from build123d import *

# Parameters (mm, degrees)
SKETCH_1_W                   = 80
SKETCH_1_H                   = 100
EXTRUDE_1_DEPTH              = 11
SKETCH_7_W                   = 15
SKETCH_7_H                   = 30
CUT_EXTRUDE_1_DEPTH          = 16
HOLE_WIZARD_M4_1_D           = 3.3
HOLE_WIZARD_M4_1_CSINK_D     = 4.05
HOLE_WIZARD_M4_1_CSINK_ANGLE = 90
FILLET_1_R                   = 20
FILLET_2_R                   = 2
SKETCH_9_W                   = 6
SKETCH_9_H                   = 35
CUT_EXTRUDE_2_DEPTH          = 11
SKETCH_11_R                  = 3
CUT_EXTRUDE_4_DEPTH          = 15
SKETCH_12_R                  = 3.43
CUT_EXTRUDE_5_DEPTH          = 3.9
CUT_EXTRUDE_6_DEPTH          = 5.4
CUT_EXTRUDE_7_DEPTH          = 14
SKETCH_15_R                  = 1.9
CUT_EXTRUDE_8_DEPTH          = 14
FILLET_4_R                   = 0.12
FILLET_5_R                   = 1


with BuildPart() as part:
    # 草图1 → 凸台-拉伸1 (new body)
    with BuildSketch(Plane.XY):
        Rectangle(SKETCH_1_W, SKETCH_1_H)
    extrude(amount=EXTRUDE_1_DEPTH)

    # 草图7 → 切除-拉伸1 (cut)
    with BuildSketch(Plane.XY.offset(11)):
        with Locations((0, 35)):
            Rectangle(SKETCH_7_W, SKETCH_7_H)
    extrude(amount=-CUT_EXTRUDE_1_DEPTH, mode=Mode.SUBTRACT)

    # M4 螺纹孔1 (through all)
    with Locations(Plane(origin=(13.5, 24.75, 0), x_dir=(-1, 0, 0), z_dir=(0, 0, -1))):
        with Locations((0, 0), (27, 0), (41.5, -49.5), (-14.5, -49.5)):
            CounterSinkHole(HOLE_WIZARD_M4_1_D / 2, HOLE_WIZARD_M4_1_CSINK_D / 2, counter_sink_angle=HOLE_WIZARD_M4_1_CSINK_ANGLE)

    # 圆角1
    fillet_1_edges = [part.edges().sort_by_distance(p)[0] for p in [
        (-40, 50, 5.5),
        (40, 50, 5.5),
    ]]
    fillet(fillet_1_edges, radius=FILLET_1_R)

    # 圆角2
    fillet_2_edges = [part.edges().sort_by_distance(p)[0] for p in [
        (-7.5, 20, 5.5),
        (-7.5, 50, 5.5),
        (7.5, 50, 5.5),
        (7.5, 20, 5.5),
        (40, -50, 5.5),
        (-40, -50, 5.5),
    ]]
    fillet(fillet_2_edges, radius=FILLET_2_R)

    # 草图9 → 切除-拉伸2 (cut)
    with BuildSketch(Plane.XY):
        with Locations((37, 0)):
            Rectangle(SKETCH_9_W, SKETCH_9_H)
        with Locations((-37, 0)):
            Rectangle(SKETCH_9_W, SKETCH_9_H)
    extrude(amount=CUT_EXTRUDE_2_DEPTH, mode=Mode.SUBTRACT)

    # 草图11 → 切除-拉伸4 (cut)
    with BuildSketch(Plane.XY):
        with Locations((-22.273863607, 38.273863607)):
            Circle(SKETCH_11_R)
        with Locations((22.273863607, 38.273863607)):
            Circle(SKETCH_11_R)
        with Locations((22.273863607, -6.273863607)):
            Circle(SKETCH_11_R)
        with Locations((-22.273863607, -6.273863607)):
            Circle(SKETCH_11_R)
    extrude(amount=CUT_EXTRUDE_4_DEPTH, mode=Mode.SUBTRACT)

    # 草图12 → 切除-拉伸5 (cut)
    with BuildSketch(Plane.XY):
        with Locations((13.5, 24.75)):
            Circle(SKETCH_12_R)
        with Locations((28, -24.75)):
            Circle(SKETCH_12_R)
        with Locations(Location((-28, -24.75, 0), (0, 0, 180))):
            Circle(SKETCH_12_R)
        with Locations(Location((-13.5, 24.75, 0), (0, 0, 180))):
            Circle(SKETCH_12_R)
    extrude(amount=CUT_EXTRUDE_5_DEPTH, mode=Mode.SUBTRACT)

    # 草图13 → 切除-拉伸6 (cut)
    with BuildSketch(Plane.XY.offset(11)):
        Polygon((-19.42752678, 33.343863607), (-16.581189953, 38.273863607), (-19.42752678, 43.203863607), (-25.120200434, 43.203863607), (-27.966537262, 38.273863607), (-25.120200434, 33.343863607), align=None)
        Polygon((-19.42752678, -11.203863607), (-16.581189953, -6.273863607), (-19.42752678, -1.343863607), (-25.120200434, -1.343863607), (-27.966537262, -6.273863607), (-25.120200434, -11.203863607), align=None)
        Polygon((25.120200434, -11.203863607), (19.42752678, -11.203863607), (16.581189953, -6.273863607), (19.42752678, -1.343863607), (25.120200434, -1.343863607), (27.966537262, -6.273863607), align=None)
        Polygon((25.120200434, 33.343863607), (19.42752678, 33.343863607), (16.581189953, 38.273863607), (19.42752678, 43.203863607), (25.120200434, 43.203863607), (27.966537262, 38.273863607), align=None)
    extrude(amount=-CUT_EXTRUDE_6_DEPTH, mode=Mode.SUBTRACT)

    # 草图14 → 切除-拉伸7 (cut)
    with BuildSketch(Plane(origin=(0, 0, 0), x_dir=(-1, 0, 0), z_dir=(0, 0, -1))):
        with BuildLine():
            Line((-42.281489137, -24.75), (-32.43, -24.75))
            ThreePointArc((-32.43, -24.75), (-32.229391744, -26.068008147), (-31.645735677, -27.266646852))
            ThreePointArc((-31.645735677, -27.266646852), (-30.468858677, -28.074682546), (-29.053003561, -27.892157349))
            Line((-29.053003561, -27.892157349), (-24.314984036, -25.345764556))
            ThreePointArc((-24.314984036, -25.345764556), (-23.168394001, -24.901228134), (-21.947979567, -24.75))
            Line((-21.947979567, -24.75), (21.947979567, -24.75))
            ThreePointArc((21.947979567, -24.75), (23.168394001, -24.901228134), (24.314984036, -25.345764556))
            Line((24.314984036, -25.345764556), (29.053003561, -27.892157349))
            ThreePointArc((29.053003561, -27.892157349), (30.468858677, -28.074682546), (31.645735677, -27.266646852))
            ThreePointArc((31.645735677, -27.266646852), (32.229391744, -26.068008147), (32.43, -24.75))
            Line((32.43, -24.75), (45.771408099, -24.75))
            Line((45.771408099, -24.75), (45.771408099, -58.548543379))
            Line((45.771408099, -58.548543379), (-42.281489137, -58.548543379))
            Line((-42.281489137, -58.548543379), (-42.281489137, -24.75))
        make_face()
    extrude(amount=-CUT_EXTRUDE_7_DEPTH, mode=Mode.SUBTRACT)

    # 草图15 → 切除-拉伸8 (cut)
    with BuildSketch(Plane.XY.offset(11)):
        with Locations((-13.5, 24.75)):
            Circle(SKETCH_15_R)
        with Locations((-28, -24.75)):
            Circle(SKETCH_15_R)
        with Locations((13.5, 24.75)):
            Circle(SKETCH_15_R)
        with Locations((28, -24.75)):
            Circle(SKETCH_15_R)
    extrude(amount=-CUT_EXTRUDE_8_DEPTH, mode=Mode.SUBTRACT)

    # 圆角4
    fillet_4_edges = [part.edges().sort_by_distance(p)[0] for p in [
        (24.660163825, -25.531277369, 1.95),
        (29.199579974, -27.963395071, 1.95),
        (-29.199579974, -27.963395071, 1.95),
        (-24.660163825, -25.531277369, 1.95),
    ]]
    fillet(fillet_4_edges, radius=FILLET_4_R)

    # 圆角5
    fillet_5_edges = [part.edges().sort_by_distance(p)[0] for p in [
        (40, -17.5, 5.5),
        (40, 17.5, 5.5),
        (-40, 17.5, 5.5),
        (-40, -17.5, 5.5),
        (40, -24.75, 5.5),
        (-40, -24.75, 5.5),
    ]]
    fillet(fillet_5_edges, radius=FILLET_5_R)


solid = part.part
The model under review builds one solid part; all positions refer to its coordinate system, in mm. A direction names the side the tool comes from. Give positions to 0.01 mm unless a question says otherwise; leave off trailing zeros. Loops run counter-clockwise (first coordinate to the right, second up) from the corner with the lowest first, then second, coordinate; pieces in that order, holes last. Notation, with made-up numbers: (-14.75, -12.75) -> (38.25, -12.75) arc R25 cw to (38.25, 18.25) -> close; hole circle Ø1 at (64.25, 37.25). An arc over 180 degrees is marked (long way). Put each result on its own line as item: value. Start each with the question number.
1. For faces 5 (the face through (-6.93, 20.6, 5.42)), 6 (the face through (-34.297, 43.986, 5.577)), 7 (the face through (18.024, -8.773, 8.338)), 8 (the face through (34, 0, 5)), 9 (the face through (-37, -17.5, 5)), list the 3-axis set-ups (+Z, -Z, +X, -X, +Y, -Y) from which the entire face can be reached by the end or side of a thin tool; tool diameter is ignored.
2. Mouldability with a two-part tool opening along Y and no side actions: class faces 1 (the face through (-22, -11.204, 8)), 2 (the face through (-8.1, 49.43, 5.42)), 3 (the face through (-7.5, 35, 6)), 4 (the face through (-24.485, 40.301, 2.761)) as released by +Y, released by -Y, zero draft, split by the parting line, or undercut.
3. We need section B-B on x = -13.5. State the section outline as (y, z) points.
4. Wall thickness on probe 1 along Y at (x, z) = (-19.5, 9); probe 2 along Y at (x, z) = (13.5, 7.5); probe 3 along X at (y, z) = (36, 3.25): over which ranges is each line inside the solid? List them lowest first.
5. We need section D-D on x = 23. State the section outline as (y, z) points.
6. We need section C-C on y = -8. State the section outline as (x, z) points.
7. Clearance check with flat-ended pins moving along their axes: P1, Ø6, axis at x = 21, z = 8.5, coming from the +Y side; P2, Ø1.5, axis at y = 10, z = 4.5, coming from the +X side; P3, Ø6, axis at x = 0, z = 2, coming from the +Y side; P4, Ø6, axis at x = -23, z = 8, coming from the -Y side. State where each tip first meets the part, or that it passes through.
8. We need section A-A on y = 24.75. State the section outline as (x, z) points, then the cut area to 3 significant figures.
Determined:
1. face 5: +Z, -Z, +Y
1. face 6: +Z, -Z, -X, +Y
1. face 7: +Z
1. face 8: +Z, -Z, +X
1. face 9: +Z, -Z, -X
2. face 1: undercut
2. face 2: released by +Y
2. face 3: zero draft
2. face 4: undercut
3. outline: (-24.75, 0) -> (21.32, 0) -> (21.32, 3.9) -> (22.85, 3.9) -> (22.85, 11) -> (-24.75, 11) -> close; (26.65, 3.9) -> (28.18, 3.9) -> (28.18, 0) -> (50, 0) -> (50, 11) -> (26.65, 11) -> close
4. probe 1: -24.75 to -11.2, -1.34 to 33.34, 43.2 to 50
4. probe 2: -24.75 to 22.85, 26.65 to 50
4. probe 3: -39.08 to -24.23, -20.32 to -7.5, 7.5 to 20.32, 24.23 to 39.08
5. outline: (-24.86, 0) -> (-9.18, 0) -> (-9.18, 5.6) -> (-11.2, 5.6) -> (-11.2, 11) -> (-24.86, 11) -> close; (-3.36, 0) -> (35.36, 0) -> (35.36, 5.6) -> (33.34, 5.6) -> (33.34, 11) -> (-1.34, 11) -> (-1.34, 5.6) -> (-3.36, 5.6) -> close; (41.18, 0) -> (49.77, 0) -> (49.77, 11) -> (43.2, 11) -> (43.2, 5.6) -> (41.18, 5.6) -> close
6. outline: (-34, 0) -> (-24.73, 0) -> (-24.73, 5.6) -> (-26.97, 5.6) -> (-26.97, 11) -> (-34, 11) -> close; (-19.82, 0) -> (19.82, 0) -> (19.82, 5.6) -> (17.58, 5.6) -> (17.58, 11) -> (-17.58, 11) -> (-17.58, 5.6) -> (-19.82, 5.6) -> close; (24.73, 0) -> (34, 0) -> (34, 11) -> (26.97, 11) -> (26.97, 5.6) -> (24.73, 5.6) -> close
7. P1: y = 50
7. P2: x = 34
7. P3: y = 20
7. P4: y = -26.25
8. outline: (-40, 0) -> (-16.93, 0) -> (-16.93, 3.9) -> (-15.4, 3.9) -> (-15.4, 11) -> (-40, 11) -> close; (-11.6, 3.9) -> (-10.07, 3.9) -> (-10.07, 0) -> (-7.5, 0) -> (-7.5, 11) -> (-11.6, 11) -> close; (7.5, 0) -> (10.07, 0) -> (10.07, 3.9) -> (11.6, 3.9) -> (11.6, 11) -> (7.5, 11) -> close; (15.4, 3.9) -> (16.93, 3.9) -> (16.93, 0) -> (40, 0) -> (40, 11) -> (15.4, 11) -> close
8. area: 608 mm^2
